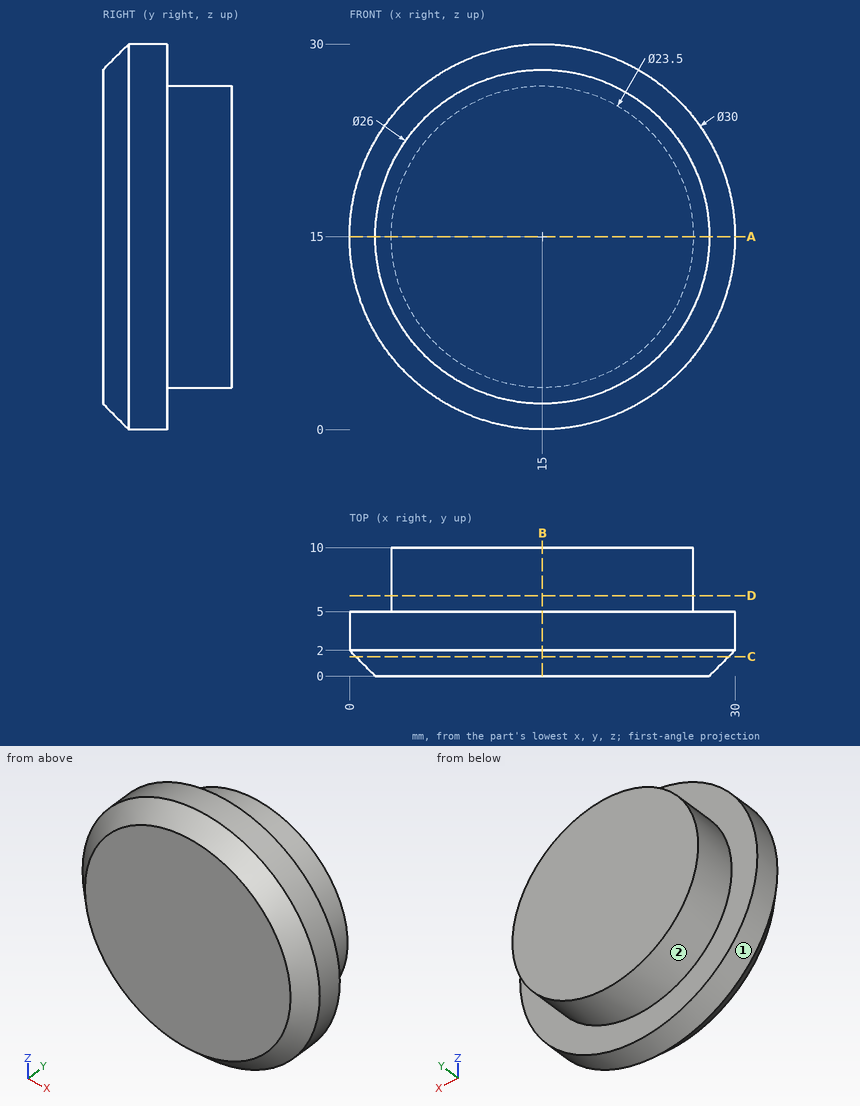
Part print with two shaded views. Sizes in mm from the minimum x, y, z corner. A direction names the side the tool comes from. Coordinates: 2 decimals unless noted, no trailing zeros. Write each loop counter-clockwise with the first axis right and the second up, starting at its lowest first coordinate (ties: lowest second). Pieces come first, ordered by that corner, then holes. Notation, with made-up numbers: M -8,26 L 42,26 A8 ccw 42,41 Z; hole C -27,-9 d7. An arc over 180 degrees is marked long. Return JSON: item names as keys, results as strings.
Item 1: Slice it at A-A, the plane z = 15. Write the cut outline in (x, y), and give its area (4 significant figures).
Findings below:
{"outline": "M 0,2 L 2,0 L 28,0 L 30,2 L 30,5 L 26.75,5 L 26.75,10 L 3.25,10 L 3.25,5 L 0,5 Z", "area": "263.5 mm2"}
Item 2: Which spindle directions (+Z, -Z, +X, -X, +Y, -Y) get a long thin tool onto all of the face, cutting with end or side? Do the marked faces 1 and 2. Say none if no direction does.
Findings below:
{"face 1": "+Y, -Y", "face 2": "+Y"}
Item 3: Drop flat-ended pins along their axis: pin 1 Ø2 at (y, z) = (5, 24.5) entering from +X; pin 2 Ø3 at (x, y) = (7, 1.5) entering from -Z; pin 3 Ø4 at (y, z) = (8, 23.5) entering from -X. Give the stop position or say it passes through.
Findings below:
{"pin 1": "stops at x = 27.36", "pin 2": "stops at z = 1.52", "pin 3": "stops at x = 5.21"}
Item 4: Probe line 1 (X direction, y = 7, z = 14.75); line 2 (Y direction, x = 11, z = 27); line 3 (X direction, y = 5.5, z = 12). List the from-to ranges inside material, lowest first. Write a range as from..to.
Findings below:
{"line 1": "x = 3.25..26.75", "line 2": "y = 0..5", "line 3": "x = 3.64..26.36"}
Item 5: Slice it at D-D, the plane y = 6.25. Write the cut outline in (x, z), and give its area (3 significant figures).
Findings below:
{"outline": "C 15,15 d23.5", "area": "434 mm2"}
Item 6: Slice it at B-B, the plane x = 15. Write the cut outline in (y, z).
Findings below:
{"outline": "M 0,2 L 2,0 L 5,0 L 5,3.25 L 10,3.25 L 10,26.75 L 5,26.75 L 5,30 L 2,30 L 0,28 Z"}
Item 7: Slice it at C-C, the plane y = 1.5. Write the cut outline in (x, z).
Findings below:
{"outline": "C 15,15 d29"}
